Autodesk Fusion 360 part; units mm, degrees
sketch "Exact underside rim - R3 desk, R1 shoulders, square chair" plane through (0, 0, 0) normal (0, 0, 1) x (1, 0, 0)
  line L0 (-75.3, 35.6) -> (-24, 35.6)
  arc A0 (-24, 35.6) -> (-23, 36.6) centre (-24, 36.6) ccw
  line L1 (-23, 36.6) -> (-23, 37.6)
  arc A1 (-23, 37.6) -> (-24, 38.6) centre (-24, 37.6) ccw
  line L2 (-24, 38.6) -> (-30, 38.6)
  arc A2 (-33, 41.6) -> (-30, 38.6) centre (-30, 41.6) ccw
  line L3 (-33, 41.6) -> (-33, 61.6)
  arc A3 (-30, 64.6) -> (-33, 61.6) centre (-30, 61.6) ccw
  line L4 (-30, 64.6) -> (26, 64.6)
  arc A4 (29, 61.6) -> (26, 64.6) centre (26, 61.6) ccw
  line L5 (29, 61.6) -> (29, -61.6)
  arc A5 (26, -64.6) -> (29, -61.6) centre (26, -61.6) ccw
  line L6 (26, -64.6) -> (-30, -64.6)
  arc A6 (-33, -61.6) -> (-30, -64.6) centre (-30, -61.6) ccw
  line L7 (-33, -61.6) -> (-33, -41.6)
  arc A7 (-30, -38.6) -> (-33, -41.6) centre (-30, -41.6) ccw
  line L8 (-30, -38.6) -> (-24, -38.6)
  arc A8 (-24, -38.6) -> (-23, -37.6) centre (-24, -37.6) ccw
  line L9 (-23, -37.6) -> (-23, -36.6)
  arc A9 (-23, -36.6) -> (-24, -35.6) centre (-24, -36.6) ccw
  line L10 (-24, -35.6) -> (-75.3, -35.6)
  line L11 (-75.3, -35.6) -> (-75.3, 35.6)
extrude "Plate - exact flush rim and flat floor" add sketch "Exact underside rim - R3 desk, R1 shoulders, square chair" along normal blind 4.5
sketch "M2 through holes" plane through (0, 0, 0) normal (0, 0, 1) x (1, 0, 0)
  circle A0 centre (-30, -61.6) radius 1.15
  circle A1 centre (26, -61.6) radius 1.15
  circle A2 centre (-30, 61.6) radius 1.15
  circle A3 centre (26, 61.6) radius 1.15
  dimension "d8" = 2.3
  dimension "d9" = 2.3
  dimension "d10" = 2.3
  dimension "d11" = 2.3
extrude "M2 through holes (1)" cut sketch "M2 through holes" along normal blind 4.5
sketch "Recessed M2 heads on floor side" plane through (0, 0, 0) normal (0, 0, 1) x (1, 0, 0)
  circle A0 centre (-30, -61.6) radius 2.15
  circle A1 centre (26, -61.6) radius 2.15
  circle A2 centre (-30, 61.6) radius 2.15
  circle A3 centre (26, 61.6) radius 2.15
  dimension "d14" = 4.3
  dimension "d15" = 4.3
  dimension "d16" = 4.3
  dimension "d17" = 4.3
extrude "Recessed M2 heads on floor side (1)" cut sketch "Recessed M2 heads on floor side" along normal blind 2.3
equation "plate_thickness = 4.5 mm"
equation "clearance = 0.3 mm"
equation "screw_diameter = 2 mm"
equation "screw_head_diameter = 4 mm"
equation "screw_head_height = 2 mm"
equation "d6 = plate_thickness"
equation "d8 = screw_diameter + clearance"
equation "d9 = screw_diameter + clearance"
equation "d10 = screw_diameter + clearance"
equation "d11 = screw_diameter + clearance"
equation "d12 = plate_thickness"
equation "d14 = screw_head_diameter + clearance"
equation "d15 = screw_head_diameter + clearance"
equation "d16 = screw_head_diameter + clearance"
equation "d17 = screw_head_diameter + clearance"
equation "d18 = screw_head_height + clearance"
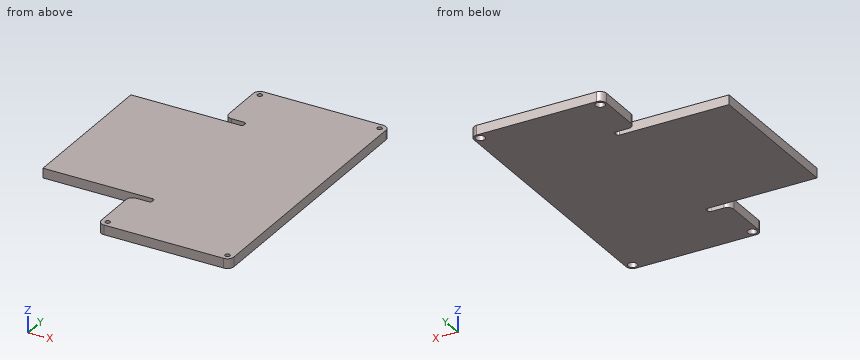
The listing builds one solid part. Answer for the finished solid, in the listing's coordinates (mm). Round coordinates to 2 decimals unless told otherwise and drop trailing zeros. Order: outer loops, then holes, each group sorted by start corner. A loop starts at its lowest first (then second) coordinate and runs counter-clockwise, first axis right, second up. Notation, with made-up numbers: (82, 40.5) - (128, 40.5) arc R29 ccw to (128, 71.5) - close; hole circle Ø10 at (45.5, -21). An arc over 180 degrees is marked (long way). Put each result on its own line as item: value. Start each with the question number.
(1) Given P1, Ø1.3, axis at x = -29, y = -62.5, coming from the -Z side; P2, Ø1.8, axis at x = 26, y = 61.6, coming from the +Z side; P3, Ø0.8, axis at y = -37, z = 2, coming from the -X side, each flat-ended and moving along its own axis, determine where each tip first touches the part or whether it passes through.
(2) Find section A-A (z = 1.05). Give the vertices of the cut face in (x, y), plus the area to 3 significant figures.
(3) Find section B-B (x = -52). Give the vertices of the cut face in (y, z).
(4) Straight lines are drawn through the part: probe 1 along X at (y, z) = (-61.6, 3.4); probe 2 along Y at (x, z) = (26, 3.3); probe 3 along Y at (x, z) = (-30, 1.05). For each, find the intervals that lie inside material, in ascending order. Write a range as from..to.
(5) Find section C-C (y = 56.5). Give the vertices of the cut face in (x, z).
Reply:
1. P1: z = 2.3
1. P2: through
1. P3: x = -23
2. outline: (-75.3, -35.6) - (-24, -35.6) arc R1 cw to (-23, -36.6) - (-23, -37.6) arc R1 cw to (-24, -38.6) - (-30, -38.6) arc R3 ccw to (-33, -41.6) - (-33, -61.6) arc R3 ccw to (-30, -64.6) - (26, -64.6) arc R3 ccw to (29, -61.6) - (29, 61.6) arc R3 ccw to (26, 64.6) - (-30, 64.6) arc R3 ccw to (-33, 61.6) - (-33, 41.6) arc R3 ccw to (-30, 38.6) - (-24, 38.6) arc R1 cw to (-23, 37.6) - (-23, 36.6) arc R1 cw to (-24, 35.6) - (-75.3, 35.6) - close; hole circle Ø4.3 at (-30, -61.6); hole circle Ø4.3 at (-30, 61.6); hole circle Ø4.3 at (26, -61.6); hole circle Ø4.3 at (26, 61.6)
2. area: 10,900 mm^2
3. outline: (-35.6, 0) - (35.6, 0) - (35.6, 4.5) - (-35.6, 4.5) - close
4. probe 1: -33..-31.15, -28.85..24.85, 27.15..29
4. probe 2: -64.6..-62.75, -60.45..60.45, 62.75..64.6
4. probe 3: -64.6..-63.75, -59.45..-38.6, -35.6..35.6, 38.6..59.45, 63.75..64.6
5. outline: (-33, 0) - (29, 0) - (29, 4.5) - (-33, 4.5) - close
